Autodesk Inventor part; units mm, degrees
ref_plane "YZ Plane" through (0, 0, 0) normal (1, 0, 0) x (0, 1, 0)
ref_plane "XZ Plane" through (0, 0, 0) normal (0, 1, 0) x (-1, 0, 0)
ref_plane "XY Plane" through (0, 0, 0) normal (0, 0, 1) x (1, 0, 0)
sketch "Sketch1" plane through (0, 0, 0) normal (1, 0, 0) x (0, 1, 0)
  circle A0 centre (0, 0) radius 11
  line L0 (-12.7, 12.7) -> (12.7, 12.7)
  line L1 (12.7, 12.7) -> (12.7, -12.7)
  line L2 (12.7, -12.7) -> (-12.7, -12.7)
  line L3 (-12.7, -12.7) -> (-12.7, 12.7)
  line L4 (-12.7, 12.7) -> (12.7, -12.7) construction
  line L5 (12.7, 12.7) -> (-12.7, -12.7) construction
  line L6 (-9.525, 9.525) -> (9.525, 9.525) construction
  line L7 (9.525, 9.525) -> (9.525, -9.525) construction
  line L8 (9.525, -9.525) -> (-9.525, -9.525) construction
  line L9 (-9.525, -9.525) -> (-9.525, 9.525) construction
  line L10 (-9.525, 9.525) -> (9.525, -9.525) construction
  line L11 (9.525, 9.525) -> (-9.525, -9.525) construction
  circle A1 centre (9.525, 9.525) radius 1.7526
  circle A2 centre (-9.525, 9.525) radius 1.7526
  circle A3 centre (-9.525, -9.525) radius 1.7526
  circle A4 centre (9.525, -9.525) radius 1.7526
  dimension "d0" = 22
  dimension "d1" = 25.4
  dimension "d2" = 25.4
  dimension "d3" = 19.05
  dimension "d4" = 19.05
  dimension "d5" = 3.5052
  dimension "d8" = 360
extrude "Extrusion1" add sketch "Sketch1" along normal blind 16.8
sketch "Sketch2" plane through (0, 12.7, 12.7) normal (0, 1, 0) x (1, 0, 0)
  circle A0 centre (12.0375, -3.175) radius 4.7625
  circle A1 centre (12.0375, -3.175) radius 3.175
  line L0 (0, 0) -> (16.8, 0)
  line L1 (16.8, 25.4) -> (16.8, 0)
  line L2 (0, 12.7) -> (16.8, 12.7) construction
  line L3 (8.6699, -6.5426) -> (2.1273, 0)
  line L4 (16.8, -3.175) -> (16.8, 0)
  circle A2 centre (12.0375, 28.575) radius 4.7625
  circle A3 centre (12.0375, 28.575) radius 3.175
  line L5 (0, 25.4) -> (16.8, 25.4)
  line L6 (8.6699, 31.9426) -> (2.1273, 25.4)
  line L7 (16.8, 28.575) -> (16.8, 25.4)
  dimension "d12" = 9.525
  dimension "d13" = 6.35
  dimension "d14" = 45
extrude "Extrusion2" add sketch "Sketch2" against normal up to surface (25.4 mm away) contours A0 L0 | L3 L0 A0 | A0 L0 L4 | A2 L5 | L7 L5 A2 | A2 L5 L6 picked at (16.1976, -2.5571) picked at (16.1976, 27.9571)
fillet "Fillet1" radius 6.35 2 edges at (2.1273, 0, -12.7) (2.1273, 0, 12.7)
thicken "Thicken1" operation cut thickness 0.254 both sides no extend neighbours no toward (0.9967573, 0, 0.0804666) faces at (15.2022, -4.2333, 16.1305)
thicken "Thicken2" operation cut thickness 0.254 both sides no extend neighbours no toward (0.9870503, 0, -0.1604113) faces at (15.1714, 4.2333, -16.3843)
properties part number "Motor Sleeve" material "UHMW, Black"
Work out the finished part from the listing and answer in its coordinate system (mm). Round coordinates to 2 decimals unless told otherwise and drop trailing zeros. Order: outer loops, then holes, each group sorted by start corner. A loop starts at its lowest first (then second) coordinate and runs counter-clockwise, first axis right, second up. Notation, with made-up numbers: M 24,-34 L 36,-34 A20 cw 36,-8 Z; hole C -31,-38.75 d1. An arc over 180 degrees is marked long. One line per item, written item: value.
Q1. Straight lines are drawn through the part: line 1 (Z direction, x = 6.25, y = -9); line 2 (Z direction, x = 2.5, y = -8.75); line 3 (Y direction, x = 12.25, z = 8). For each, find the intervals that lie inside material, in ascending order.
Derived:
line 1: -16.82 to -11.2, -7.85 to -6.32, 6.32 to 7.85, 11.2 to 16.82
line 2: -13.44 to -11.1, -7.95 to -6.67, 6.67 to 7.95, 11.1 to 13.44
line 3: -12.7 to -10.39, -8.66 to -7.55, 7.55 to 8.66, 10.39 to 12.7
Q2. Find section A-A on y = 0. Give the number of separate pieces and of enclosed holes in the cut face, then the cut area to 3 significant figures.
Derived:
separate pieces: 2
enclosed holes: 2
area: 144 mm²
Q3. Find section C-C on x = 11.25. Write down the section's boundary in (y, z) (3 decimals), then the cut area to 3 significant figures.
Derived:
outline: M -12.7,-20.572 L 12.7,-20.572 L 12.7,-19.212 L -12.7,-19.212 Z; M -12.7,-12.538 L 12.7,-12.538 L 12.7,12.538 L -12.7,12.538 Z; M -12.7,19.212 L 12.7,19.212 L 12.7,20.572 L -12.7,20.572 Z; hole C -9.525,-9.525 d3.505; hole C -9.525,9.525 d3.505; hole C 0,0 d22; hole C 9.525,-9.525 d3.505; hole C 9.525,9.525 d3.505
area: 287 mm²
Q4. Find section B-B on z = 0. Write down the section's boundary in (x, y).
Derived:
outline: M 0,-12.7 L 16.8,-12.7 L 16.8,-11 L 0,-11 Z; M 0,11 L 16.8,11 L 16.8,12.7 L 0,12.7 Z
Q5. Determine the mould class of faces 1 (the face through (13.932, 0.178, -20.244)), 2 (the face through (8.28, -2.38, 10.74)), 3 (the face through (8.282, -9.753, 7.787)), 4 (the face through (6.35, 0.18, 16.92)) for opening direction Z: released by +Z, released by -Z, zero draft, split by the parting line, or undercut.
Derived:
face 1: released by -Z
face 2: undercut
face 3: undercut
face 4: released by +Z
Q6. Flat-ended cylindrical pins translate along their axes: pin 1 (10 mm diameter, centred on y = 4, z = -1, fed in from -X); pin 2 (4 mm diameter, centred on x = 6.5, y = 2.5, fed in from -Z); pin 3 (2 mm diameter, centred on x = 9, y = 3.5, fed in from -Z). Find the tip coordinate at first contact, or state that the pin passes through.
Derived:
pin 1: through
pin 2: z = -19.07
pin 3: z = -20.18
